Work out the finished part from the listing and answer in its coordinate system (mm). Face numbers are marked on the shaded views. A direction names the side the tool comes from. Coordinates: 2 decimals unless noted, no trailing zeros. Write each loop counter-clockwise with the first axis right and the second up, starting at its lowest first coordinate (ties: lowest second). Pieces come first, ordered by that corner, then holes. Notation, with made-up numbers: (48, 88.25) - (83, 88.25) arc R14 ccw to (83, 93.25) - close; hole circle Ø9 at (40.25, 30.25). An arc over 180 degrees is marked (long way). One line per item, written item: value.
```python
from build123d import *

# Parameters (mm, degrees)
SKETCH_2_W               = 28
SKETCH_2_H               = 4.5
CUT_EXTRUDE_1_DEPTH      = 10
EXTRUDE_1_DEPTH          = 15
HOLE_WIZARD_M3_1_D       = 2.5
HOLE_WIZARD_M3_1_DEPTH   = 4
HOLE_WIZARD_M3_1_TIP     = 0.751075774
CUT_EXTRUDE_2_DEPTH      = 20
HOLE_WIZARD_M4_1_D       = 3.3
HOLE_WIZARD_M4_1_DEPTH   = 10.1
HOLE_WIZARD_M4_1_TIP     = 0.991420021
HOLE_WIZARD_M3_2_D       = 2.5
HOLE_WIZARD_M5_1_D       = 4.2
HOLE_WIZARD_M5_1_DEPTH   = 14
HOLE_WIZARD_M5_1_TIP     = 1.2618073
SKETCH_17_W              = 73.774963695
SKETCH_17_H              = 83.233292373
CUT_EXTRUDE_3_DEPTH      = 22
CUT_EXTRUDE_3_DEPTH_BACK = 22
SKETCH_18_R              = 13.4
EXTRUDE_2_DEPTH          = 2
SKETCH_19_R              = 5.75
EXTRUDE_3_DEPTH          = 6.7
SKETCH_20_R              = 1.25
CUT_EXTRUDE_4_DEPTH      = 8


with BuildPart() as part:
    # 草图1 → 旋转1 (revolve)
    with BuildSketch(Plane.XY):
        Polygon((0, 0), (4.1, 0), (4.1, 6.7), (13.4, 6.7), (13.4, 8.7), (21, 8.7), (21, 10.2), (20, 10.2), (20, 11.2), (21, 11.2), (21, 12.2), (10, 12.2), (10, 13.2), (21, 13.2), (21, 20.4), (5, 20.4), (5, 21), (21, 21), (21, 34.7), (18.3, 38.7), (3.5, 38.7), (3.5, 43.7), (0, 43.7), align=None)
    revolve(axis=Axis((0, 43.7, 0), (0, -1, 0)))

    # 草图2 → 切除-拉伸1 (cut)
    with BuildSketch(Plane.XY.offset(21)):
        with Locations((0, 16.05)):
            Rectangle(SKETCH_2_W, SKETCH_2_H)
    extrude(amount=-CUT_EXTRUDE_1_DEPTH, mode=Mode.SUBTRACT)

    # 草图3 → 凸台-拉伸1 (add)
    with BuildSketch(Plane.XY.offset(11)):
        with BuildLine():
            Line((9.185056323, 18.053194417), (9.385056323, 18.053194417))
            ThreePointArc((9.385056323, 18.053194417), (11.385056323, 16.053194417), (9.385056323, 14.053194417))
            Line((9.385056323, 14.053194417), (9.185056323, 14.053194417))
            ThreePointArc((9.185056323, 14.053194417), (7.185056323, 16.053194417), (9.185056323, 18.053194417))
        make_face()
    extrude(amount=EXTRUDE_1_DEPTH)

    # M3 螺纹孔1
    with Locations(Plane(origin=(0, 38.7, 0), x_dir=(1, 0, 0), z_dir=(0, 1, 0))):
        with Locations((-6.5, 0), (6.5, 0)):
            Hole(HOLE_WIZARD_M3_1_D / 2, depth=HOLE_WIZARD_M3_1_DEPTH)
            with Locations((0, 0, -(HOLE_WIZARD_M3_1_DEPTH + HOLE_WIZARD_M3_1_TIP / 2))):  # 118° drill point
                Cone(0, HOLE_WIZARD_M3_1_D / 2, HOLE_WIZARD_M3_1_TIP, mode=Mode.SUBTRACT)

    # 草图7 → 旋转2 (revolve)
    with BuildSketch(Plane.XY):
        Polygon((0, -54.6), (5, -54.6), (5, -30.5), (8.275, -30.5), (8.275, -29.6), (13, -29.6), (13, -27.6), (21, -27.6), (21, 8.7), (0, 8.7), align=None)
    revolve(axis=Axis((0, 8.7, 0), (0, -1, 0)))

    # 草图8 → 切除-拉伸2 (cut)
    with BuildSketch(Plane.XZ.offset(54.6)):
        with BuildLine():
            Line((-3, 4), (3, 4))
            ThreePointArc((3, 4), (0, 5), (-3, 4))
        make_face()
    extrude(amount=-CUT_EXTRUDE_2_DEPTH, mode=Mode.SUBTRACT)

    # M4 螺纹孔1
    with Locations(Plane(origin=(0, -27.6, 0), x_dir=(-1, 0, 0), z_dir=(0, -1, 0))):
        with Locations((17.5, 0), (0, -17.5), (-17.5, 0), (0, 17.5)):
            Hole(HOLE_WIZARD_M4_1_D / 2, depth=HOLE_WIZARD_M4_1_DEPTH)
            with Locations((0, 0, -(HOLE_WIZARD_M4_1_DEPTH + HOLE_WIZARD_M4_1_TIP / 2))):  # 118° drill point
                Cone(0, HOLE_WIZARD_M4_1_D / 2, HOLE_WIZARD_M4_1_TIP, mode=Mode.SUBTRACT)

    # M3 螺纹孔2 (through all)
    with Locations(Plane(origin=(0, -44.6, 4), x_dir=(1, 0, 0), z_dir=(0, 0, 1))):
        with Locations((0, 0)):
            Hole(HOLE_WIZARD_M3_2_D / 2)

    # M5 螺纹孔1
    with Locations(Plane(origin=(0, -54.6, 0), x_dir=(-1, 0, 0), z_dir=(0, -1, 0))):
        with Locations((0, 0)):
            Hole(HOLE_WIZARD_M5_1_D / 2, depth=HOLE_WIZARD_M5_1_DEPTH)
            with Locations((0, 0, -(HOLE_WIZARD_M5_1_DEPTH + HOLE_WIZARD_M5_1_TIP / 2))):  # 118° drill point
                Cone(0, HOLE_WIZARD_M5_1_D / 2, HOLE_WIZARD_M5_1_TIP, mode=Mode.SUBTRACT)

    # 草图17 → 切除-拉伸3 (cut, two sides)
    with BuildSketch(Plane(origin=(0, 0, 0), x_dir=(0, 0, -1), z_dir=(1, 0, 0))) as cut_extrude_3_sk:
        with Locations((1.792626092, -32.916646187)):
            Rectangle(SKETCH_17_W, SKETCH_17_H)
    extrude(amount=CUT_EXTRUDE_3_DEPTH, mode=Mode.SUBTRACT)
    extrude(cut_extrude_3_sk.sketch, amount=-CUT_EXTRUDE_3_DEPTH_BACK, mode=Mode.SUBTRACT)

    # 草图18 → 凸台-拉伸2 (add)
    with BuildSketch(Plane.XZ.offset(-8.7)):
        Circle(SKETCH_18_R)
    extrude(amount=EXTRUDE_2_DEPTH)

    # 草图19 → 凸台-拉伸3 (add)
    with BuildSketch(Plane.XZ.offset(-6.7)):
        Circle(SKETCH_19_R)
    extrude(amount=EXTRUDE_3_DEPTH)

    # 草图20 → 切除-拉伸4 (cut)
    with BuildSketch(Plane.XZ.offset(-8.7)):
        with Locations((-7.117891254, 15.987045509)):
            Circle(SKETCH_20_R)
        with Locations((15.987045509, 7.117891254)):
            Circle(SKETCH_20_R)
        with Locations((7.117891254, -15.987045509)):
            Circle(SKETCH_20_R)
        with Locations((-15.987045509, -7.117891254)):
            Circle(SKETCH_20_R)
    extrude(amount=-CUT_EXTRUDE_4_DEPTH, mode=Mode.SUBTRACT)


solid = part.part
```
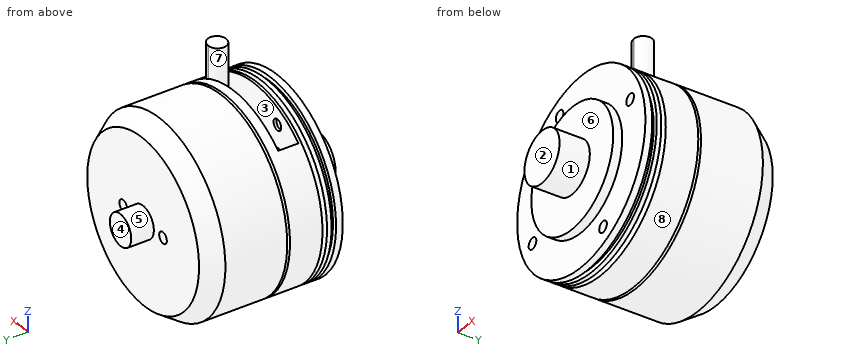
Item 1: Consider probe 1 along Y at (x, z) = (9, -8.5); probe 2 along Y at (x, z) = (-10, 13); probe 3 along Y at (x, z) = (-1, 13). Determine where each line is inside the solid, lowest interval first.
Evaluation:
probe 1: y = 6.7 to 12.2, 13.2 to 20.4, 21 to 38.7
probe 2: y = 8.7 to 12.2, 13.2 to 13.8, 18.3 to 20.4, 21 to 38.7
probe 3: y = 6.7 to 12.2, 13.2 to 13.8, 18.3 to 20.4, 21 to 38.7
Item 2: Given pin 1 (1 mm diameter, centred on y = 12.5, z = 7, fed in from +X); pin 2 (6 mm diameter, centred on x = -8.5, z = 0.5, fed in from +Y); pin 3 (2 mm diameter, centred on x = -7.12, z = 15.99, fed in from -Y), each flat-ended and moving along its own axis, determine where each tip first touches the part or whether it passes through.
Evaluation:
pin 1: stops at x = 19.94
pin 2: stops at y = 38.7
pin 3: stops at y = 18.3
Item 3: Section B-B, the plane z = -12 is taken. Give the number of separate pieces and of enclosed holes in the cut face, then the cut area to 3 significant figures.
Evaluation:
separate pieces: 3
enclosed holes: 0
area: 987 mm2
Item 4: Section A-A, the plane y = 19 is taken. Determine the outline of the cut face in (x, z).
Evaluation:
outline: circle Ø42 at (0, 0)
Item 5: Determine the mould class of the marked faces 6, 7 and 8 for opening direction X: +X half, -X half, draft (parallel to the pull), parting line (faces both ways), or undercut.
Evaluation:
face 6: draft
face 7: undercut
face 8: parting line
Item 6: Which of the six approach directions +Z, -Z, +X, -X, +Y, -Y give full straight-line access (tool end or side, diameter ignored) to the marked faces 1, 2, 3, 4 and 5?
Evaluation:
face 1: -Y
face 2: +Z, -Z, +X, -X, -Y
face 3: +Z
face 4: +Z, -Z, +X, -X, +Y
face 5: +Y
